```python
from build123d import *

# Parameters (mm, degrees)
SKETCH016_R             = 5
POCKET002_DEPTH         = 8.001
POCKET003_DEPTH         = 5.2
BODY011_PLACEMENT_ANGLE = 270


with BuildPart() as part:
    # Sketch014 → Revolution (revolve)
    with BuildSketch(Plane.XZ):
        with BuildLine():
            ThreePointArc((15, -4), (13.828427, -1.171573), (11, 0))
            Line((3.2, 0), (11, 0))
            Line((3.2, 0), (3.2, -8))
            Line((3.2, -8), (13, -8))
            Line((13, -8), (15, -6))
            Line((15, -6), (15, -4))
        make_face()
    revolve(axis=Axis((0, 0, 0), (0, 0, 1)))

    # Sketch016 → Pocket002 (cut, through all)
    with BuildSketch(Plane.XY):
        with Locations((0, 15)):
            Circle(SKETCH016_R)
        with Locations((12.990381, 7.5)):
            Circle(SKETCH016_R)
        with Locations((12.990381, -7.5)):
            Circle(SKETCH016_R)
        with Locations((0, -15)):
            Circle(SKETCH016_R)
        with Locations((-12.990381, -7.5)):
            Circle(SKETCH016_R)
        with Locations((-12.990381, 7.5)):
            Circle(SKETCH016_R)
    extrude(amount=-POCKET002_DEPTH, mode=Mode.SUBTRACT)

    # Sketch015 → Pocket003 (cut)
    with BuildSketch(Plane.XY.offset(-1.5)):
        Polygon((5.888973, 0), (2.944486, 5.1), (-2.944486, 5.1), (-5.888973, 0), (-2.944486, -5.1), (2.944486, -5.1), align=None)
    extrude(amount=-POCKET003_DEPTH, mode=Mode.SUBTRACT)


with BuildPart() as part_1:
    # Body011 placement: moved
    add(part.part.moved(Location((22.5, -70, 0))).rotate(Axis((22.5, -70, 0), (1, 0, 0)), BODY011_PLACEMENT_ANGLE))


with BuildPart() as part_2:
    # Clone006 placement: moved
    add(part_1.part.moved(Location((-45, 0, 0))))


solid = part_2.part
```
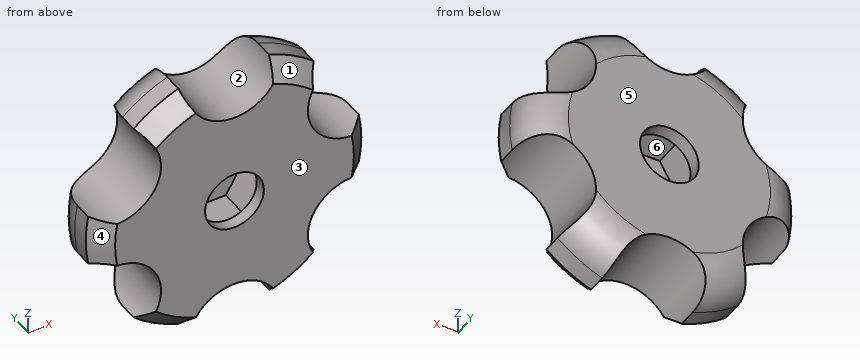
The model under review builds one solid part; all positions refer to its coordinate system, in mm. Face numbers are marked on the shaded views. A direction names the side the tool comes from. Coordinates: 2 decimals unless noted, no trailing zeros. Write each loop counter-clockwise with the first axis right and the second up, starting at its lowest first coordinate (ties: lowest second). Pieces come first, ordered by that corner, then holes.
1) To check wall thickness, follow probe 1 along Z at (x, y) = (-22.5, -77.2); probe 2 along Z at (x, y) = (-31, -75); probe 3 along Y at (x, z) = (-25.5, -4.5). State the ranges of each line that lie inside material, in increasing order.
2) We need section B-B on x = -22.5. State the section outline as (y, z) points, then the cut area to 3 significant figures.
3) We need section C-C on y = -70.5. State the section outline as (x, z) points, then the cut area to 3 significant figures.
4) Machinability: for the marked faces 5 and 6, which of the approach directions +Z, -Z, +X, -X, +Y, -Y give a long, thin tool a straight path to every point of the face, cutting with its end or side? Answer none if there is none.
5) We need section D-D on z = -7. State the section outline as (x, y) points, then the cut area to 3 significant figures.
6) The part is to be moulded in two halves that separate along X. For the marked faces 1, 2, 3 and 4, say which applies: pulls with the +X half, pulls with the -X half, needs draft (parallel to the pull), parting line crosses it, or undercut.
7) Clearance check with flat-ended pins moving along their axes: pin 1 Ø4 at (y, z) = (-74.5, -7) entering from +X; pin 2 Ø1.5 at (y, z) = (-77, 4.5) entering from +X; pin 3 Ø2 at (x, y) = (-16, -71.5) entering from +Z; pin 4 Ø11 at (x, z) = (-25.5, -1) entering from +Y. State where each tip first meets the part, or that it passes through.
8) We need section A-A on y = -74.75. State the section outline as (x, z) points, then the cut area to 3 significant figures.
Answer list:
1. probe 1: z = -10 to -3.2, 3.2 to 10
1. probe 2: z = -12.36 to -9.7, -5.3 to 5.3, 9.7 to 12.36
1. probe 3: y = -78 to -76.7, -71.5 to -70
2. outline: (-78, -10) - (-70, -10) - (-70, -3.2) - (-71.5, -3.2) - (-71.5, -5.1) - (-76.7, -5.1) - (-76.7, -3.2) - (-78, -3.2) - close; (-78, 3.2) - (-76.7, 3.2) - (-76.7, 5.1) - (-71.5, 5.1) - (-71.5, 3.2) - (-70, 3.2) - (-70, 10) - (-78, 10) - close
2. area: 89.0 mm2
3. outline: (-35.19, -2.51) arc R5 cw to (-31.02, -9.74) arc R12.94 ccw to (-26.67, -12.25) arc R5 cw to (-18.33, -12.25) arc R12.94 ccw to (-13.98, -9.74) arc R5 cw to (-9.81, -2.51) arc R12.94 ccw to (-9.81, 2.51) arc R5 cw to (-13.98, 9.74) arc R12.94 ccw to (-18.33, 12.25) arc R5 cw to (-26.67, 12.25) arc R12.94 ccw to (-31.02, 9.74) arc R5 cw to (-35.19, 2.51) arc R12.94 ccw to start; hole circle Ø6.4 at (-22.5, 0)
3. area: 391 mm2
4. face 5: +Z, -Z, +X, -X, +Y
4. face 6: none
5. outline: (-30.52, -78) - (-14.48, -78) - (-14.48, -70) - (-30.52, -70) - close
5. area: 128 mm2
6. face 1: pulls with the +X half
6. face 2: undercut
6. face 3: needs draft
6. face 4: pulls with the -X half
7. pin 1: stops at x = -13.84
7. pin 2: stops at x = -12.82
7. pin 3: stops at z = 13.38
7. pin 4: stops at y = -70
8. outline: (-37.23, -2.81) arc R5 cw to (-32.3, -11.35) arc R15 ccw to (-27.43, -14.17) arc R5 cw to (-17.57, -14.17) arc R15 ccw to (-12.7, -11.35) arc R5 cw to (-7.77, -2.81) arc R15 ccw to (-7.77, 2.81) arc R5 cw to (-12.7, 11.35) arc R15 ccw to (-17.57, 14.17) arc R5 cw to (-27.43, 14.17) arc R15 ccw to (-32.3, 11.35) arc R5 cw to (-37.23, 2.81) arc R15 ccw to start; hole (-28.39, 0) - (-25.44, -5.1) - (-19.56, -5.1) - (-16.61, 0) - (-19.56, 5.1) - (-25.44, 5.1) - close
8. area: 398 mm2
